```python
from build123d import *

# Parameters (mm, degrees)
SKETCH1_W           = 21.8
SKETCH1_H           = 12.5
BOSS_EXTRUDE1_DEPTH = 2
CUT_EXTRUDE1_REACH  = 4
SKETCH2_R           = 1.8
SKETCH3_W           = 9
SKETCH3_H           = 2
BOSS_EXTRUDE2_DEPTH = 22
SKETCH4_R           = 0.95
CUT_EXTRUDE2_DEPTH  = 13.5
SKETCH5_R           = 1.8
SKETCH5_R_2         = 1.35
BOSS_EXTRUDE3_DEPTH = 2
SKETCH6_W           = 9
SKETCH6_H           = 2
BOSS_EXTRUDE4_DEPTH = 10


with BuildPart() as part:
    # Sketch1 → Boss-Extrude1 (new body)
    with BuildSketch(Plane(origin=(0, 0, 0), x_dir=(1, 0, 0), z_dir=(0, 1, 0))):
        Rectangle(SKETCH1_W, SKETCH1_H)
    extrude(amount=BOSS_EXTRUDE1_DEPTH)

    # Sketch2 → Cut-Extrude1 (cut, up to next)
    with BuildSketch(Plane(origin=(0, 2, 0), x_dir=(1, 0, 0), z_dir=(0, 1, 0)), mode=Mode.PRIVATE) as cut_extrude1_sk1:
        with Locations((8, -3.55)):
            Circle(SKETCH2_R)
    cut_extrude1_tool1 = extrude(cut_extrude1_sk1.sketch, amount=-CUT_EXTRUDE1_REACH, mode=Mode.PRIVATE) & part.part
    add(cut_extrude1_tool1.solids().sort_by_distance((8, 2, 3.55))[0], mode=Mode.SUBTRACT)

    # Sketch3 → Boss-Extrude2 (add)
    with BuildSketch(Plane.XZ):
        with Locations((0, -5.25)):
            Rectangle(SKETCH3_W, SKETCH3_H)
    extrude(amount=BOSS_EXTRUDE2_DEPTH)

    # Sketch4 → Cut-Extrude2 (cut, through all)
    with BuildSketch(Plane(origin=(0, 0, -6.25), x_dir=(-1, 0, 0), z_dir=(0, 0, -1))):
        with Locations((0, -13.5)):
            Circle(SKETCH4_R)
        with Locations((0, -18.5)):
            Circle(SKETCH4_R)
    extrude(amount=-CUT_EXTRUDE2_DEPTH, mode=Mode.SUBTRACT)

    # Sketch5 → Boss-Extrude3 (add)
    with BuildSketch(Plane(origin=(0, 2, 0), x_dir=(1, 0, 0), z_dir=(0, 1, 0))):
        with Locations((8, -3.55)):
            Circle(SKETCH5_R)
        with Locations((8, -3.55)):
            Circle(SKETCH5_R_2, mode=Mode.SUBTRACT)
    extrude(amount=-BOSS_EXTRUDE3_DEPTH)

    # Sketch6 → Boss-Extrude4 (add)
    with BuildSketch(Plane.XZ):
        with Locations((0, -3.25)):
            Rectangle(SKETCH6_W, SKETCH6_H)
    extrude(amount=BOSS_EXTRUDE4_DEPTH)


solid = part.part
```
The model under review builds one solid part; all positions refer to its coordinate system, in mm. A direction names the side the tool comes from. Give positions to 0.01 mm unless a question says otherwise; leave off trailing zeros. Write each loop counter-clockwise with the first axis right and the second up, starting at its lowest first coordinate (ties: lowest second). Pieces come first, ordered by that corner, then holes. Notation, with made-up numbers: (-13.5, 35.5) -> (39.5, 35.5) arc R27 cw to (39.5, 59.5) -> close; hole circle Ø4 at (-15.75, 68). An arc over 180 degrees is marked (long way). Put each result on its own line as item: value.
(1) We need section D-D, the plane z = -5.25. Give the boundary of the cut face in (x, y), and give its area (3 significant figures).
Results are:
outline: (-10.9, 0) -> (-4.5, 0) -> (-4.5, -22) -> (4.5, -22) -> (4.5, 0) -> (10.9, 0) -> (10.9, 2) -> (-10.9, 2) -> close; hole circle Ø1.9 at (0, -18.5); hole circle Ø1.9 at (0, -13.5)
area: 236 mm²
(2) We need section A-A, the plane x = 8. Give the boundary of the cut face in (y, z), and give its area (3 significant figures).
Results are:
outline: (0, -6.25) -> (2, -6.25) -> (2, 2.2) -> (0, 2.2) -> close; (0, 4.9) -> (2, 4.9) -> (2, 6.25) -> (0, 6.25) -> close
area: 19.6 mm²
(3) We need section B-B, the plane z = 3.55. Give the boundary of the cut face in (x, y).
Results are:
outline: (-10.9, 0) -> (6.65, 0) -> (6.65, 2) -> (-10.9, 2) -> close; (9.35, 0) -> (10.9, 0) -> (10.9, 2) -> (9.35, 2) -> close
(4) For pin 1 Ø10 at (x, y) = (-1, -17.5) entering from +Z; pin 2 Ø5 at (x, z) = (4.5, 2) entering from -Y; pin 3 Ø1.1 at (x, y) = (0, -18.5) entering from +Z; pin 4 Ø5 at (x, y) = (-5, -11.5) entering from +Z, all flat-tipped, find the tip position at first contact; note any pin that passes through.
Results are:
pin 1: z = -4.25
pin 2: y = 0
pin 3: through
pin 4: z = -2.25
(5) The part is to be moulded in two halves that separate along Y. For faces 1 (the flat face through (0, -10, -3)), 2 (the flat face through (0, 2, 0)), 3 (the flat face through (0, 1, 6.25)), 4 (the cylindrical face through (0.206, -19.427, -5.264)), say which applies: pulls with the +Y half, pulls with the -Y half, needs draft (parallel to the pull), parting line crosses it, or undercut.
Results are:
face 1: pulls with the -Y half
face 2: pulls with the +Y half
face 3: needs draft
face 4: undercut
(6) Tool access review of faces 5 (the flat face through (4.5, -8, -5)), 6 (the flat face through (0, -5, -2.25)), 7 (the cylindrical face through (9.247, 1.014, 4.067)), 8 (the flat face through (-4.5, -8, -5)): name each direction out of +Z, -Z, +X, -X, +Y, -Y from which nothing blocks a thin tool from reaching the whole face with its end or side.
Results are:
face 5: +Z, -Z, +X, -Y
face 6: +Z, +X, -X, -Y
face 7: +Y, -Y
face 8: +Z, -Z, -X, -Y
(7) To check wall thickness, follow probe 1 along Y at (x, z) = (0, -4.8); probe 2 along X at (y, z) = (0.85, 3.55); probe 3 along Z at (x, y) = (8, 0.55). State the ranges of each line that lie inside material, in increasing order. Write a range as from..to.
Results are:
probe 1: -22..-19.45, -17.55..-14.45, -12.55..2
probe 2: -10.9..6.65, 9.35..10.9
probe 3: -6.25..2.2, 4.9..6.25
(8) We need section C-C, the plane x = 0. Give the boundary of the cut face in (y, z).
Results are:
outline: (-22, -6.25) -> (-19.45, -6.25) -> (-19.45, -4.25) -> (-22, -4.25) -> close; (-17.55, -6.25) -> (-14.45, -6.25) -> (-14.45, -4.25) -> (-17.55, -4.25) -> close; (-12.55, -6.25) -> (2, -6.25) -> (2, 6.25) -> (0, 6.25) -> (0, -2.25) -> (-10, -2.25) -> (-10, -4.25) -> (-12.55, -4.25) -> close
